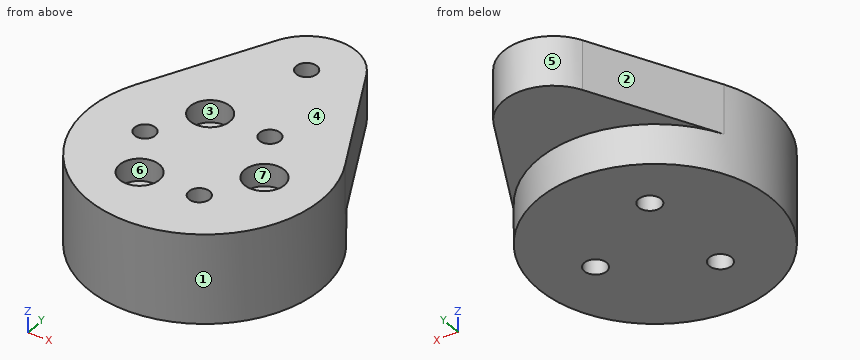
from build123d import *

# Parameters (mm, degrees)
SKETCH1_R           = 23.5
BOSS_EXTRUDE1_DEPTH = 18
BOSS_EXTRUDE2_START = -10
BOSS_EXTRUDE2_DEPTH = 10
SKETCH8_R           = 2.25
CUT_EXTRUDE3_DEPTH  = 50.761933242
SKETCH9_R           = 4
CUT_EXTRUDE4_DEPTH  = 4.5
SKETCH10_R          = 2.1
CUT_EXTRUDE5_DEPTH  = 5.7


with BuildPart() as part:
    # Sketch1 → Boss-Extrude1 (new body)
    with BuildSketch(Plane.XY):
        Circle(SKETCH1_R)
    extrude(amount=BOSS_EXTRUDE1_DEPTH)

    # Sketch7 → Boss-Extrude2 (add)
    with BuildSketch(Plane.XY.offset(18).offset(BOSS_EXTRUDE2_START)):
        with BuildLine():
            ThreePointArc((0, 23.5), (12.323503966, 20.00952898), (20.986171042, 10.575))
            Line((20.986171042, 10.575), (8.93028555, 34.5))
            ThreePointArc((8.93028555, 34.5), (0, 40), (-8.93028555, 34.5))
            Line((-8.93028555, 34.5), (-20.986171042, 10.575))
            ThreePointArc((-20.986171042, 10.575), (-12.323503966, 20.00952898), (0, 23.5))
        make_face()
    extrude(amount=BOSS_EXTRUDE2_DEPTH)

    # Sketch8 → Cut-Extrude3 (cut, through all)
    with BuildSketch(Plane.XY.offset(18)):
        with Locations((12, 0)):
            Circle(SKETCH8_R)
        with Locations((-6, -10.392304845)):
            Circle(SKETCH8_R)
        with Locations((-6, 10.392304845)):
            Circle(SKETCH8_R)
    extrude(amount=-CUT_EXTRUDE3_DEPTH, mode=Mode.SUBTRACT)

    # Sketch9 → Cut-Extrude4 (cut)
    with BuildSketch(Plane.XY.offset(18)):
        with Locations((-6, 10.392304845)):
            Circle(SKETCH9_R)
        with Locations((12, 0)):
            Circle(SKETCH9_R)
        with Locations((-6, -10.392304845)):
            Circle(SKETCH9_R)
    extrude(amount=-CUT_EXTRUDE4_DEPTH, mode=Mode.SUBTRACT)

    # Sketch10 → Cut-Extrude5 (cut)
    with BuildSketch(Plane.XY.offset(18)):
        with Locations((0, 30)):
            Circle(SKETCH10_R)
        with Locations((12, 0)):
            Circle(SKETCH10_R)
        with Locations((6, -10.392304845)):
            Circle(SKETCH10_R)
        with Locations((-6, -10.392304845)):
            Circle(SKETCH10_R)
        with Locations((-12, 0)):
            Circle(SKETCH10_R)
        with Locations((-6, 10.392304845)):
            Circle(SKETCH10_R)
        with Locations((6, 10.392304845)):
            Circle(SKETCH10_R)
    extrude(amount=-CUT_EXTRUDE5_DEPTH, mode=Mode.SUBTRACT)


solid = part.part
Work out the finished part from the listing and answer in its coordinate system (mm). Face numbers are marked on the shaded views. A direction names the side the tool comes from. Give positions to 0.01 mm unless a question says otherwise; leave off trailing zeros. Order: outer loops, then holes, each group sorted by start corner. A loop starts at its lowest first (then second) coordinate and runs counter-clockwise, first axis right, second up. Notation, with made-up numbers: (-1, 40) - (4, 40) arc R20 ccw to (4, 60) - close; hole circle Ø10 at (50, 13.25). An arc over 180 degrees is marked (long way). Answer as CSV lines item,"result". Start each with the question number.
Q1. For the marked faces 1, 2 and 3, determine the directions among +Z, -Z, +X, -X, +Y, -Y from which every point of the face is accessible in a straight line to the end or side of a thin tool.
Q2. The part is cut by section C-C (x = 12). Write down the section's boundary in (y, z).
Q3. Given pin 1 Ø4 at (y, z) = (-8, 2) entering from +X; pin 2 Ø6 at (x, y) = (-6, -10.39) entering from +Z; pin 3 Ø1.5 at (y, z) = (-16.5, 2.5) entering from +X, each flat-ended and moving along its own axis, determine where each tip first touches the part or whether it passes through.
Q4. The part is cut by section D-D (y = 30). Write down the section's boundary in (x, z), then the cut area to 3 significant figures.
Q5. The mould has two halves that part along Y. Classify the marked faces 4, 5, 6 and 7: +Y half, -Y half, draft (parallel to the pull), parting line (faces both ways), or undercut.
Q6. The part is cut by section B-B (x = -6). Write down the section's boundary in (y, z).
Q7. Find the intervals of material crossed by L1, parallel to Y at x = -6, z = 15.3; L2, parallel to Y at x = -6, z = 6.5; L3, parallel to Y at x = -12, z = 16.5, in increasing order. Write a range as [from, to].
Q8. The part is cut by section A-A (y = 0). Write down the section's boundary in (x, z).
Check result:
1,face 1,"-Z"
1,face 2,"+Z, -Z, -X, +Y"
1,face 3,"+Z"
2,outline,"(-20.21, 0) - (-2.25, 0) - (-2.25, 13.5) - (-4, 13.5) - (-4, 18) - (-20.21, 18) - close; (2.25, 0) - (20.21, 0) - (20.21, 8) - (28.41, 8) - (28.41, 18) - (4, 18) - (4, 13.5) - (2.25, 13.5) - close"
3,pin 1,"stops at x = 22.72"
3,pin 2,"stops at z = 13.5"
3,pin 3,"stops at x = 17.44"
4,outline,"(-11.2, 8) - (11.2, 8) - (11.2, 18) - (2.1, 18) - (2.1, 12.3) - (-2.1, 12.3) - (-2.1, 18) - (-11.2, 18) - close"
4,area,"200 mm²"
5,face 4,"draft"
5,face 5,"+Y half"
5,face 6,"undercut"
5,face 7,"undercut"
6,outline,"(-22.72, 0) - (-12.64, 0) - (-12.64, 13.5) - (-14.39, 13.5) - (-14.39, 18) - (-22.72, 18) - close; (-8.14, 0) - (8.14, 0) - (8.14, 13.5) - (6.39, 13.5) - (6.39, 18) - (-6.39, 18) - (-6.39, 13.5) - (-8.14, 13.5) - close; (12.64, 0) - (22.72, 0) - (22.72, 8) - (38, 8) - (38, 18) - (14.39, 18) - (14.39, 13.5) - (12.64, 13.5) - close"
7,L1,"y = [-22.72, -14.39], [-6.39, 6.39], [14.39, 38]"
7,L2,"y = [-22.72, -12.64], [-8.14, 8.14], [12.64, 22.72]"
7,L3,"y = [-20.21, -2.1], [2.1, 28.41]"
8,outline,"(-23.5, 0) - (9.75, 0) - (9.75, 13.5) - (8, 13.5) - (8, 18) - (-9.9, 18) - (-9.9, 12.3) - (-14.1, 12.3) - (-14.1, 18) - (-23.5, 18) - close; (14.25, 0) - (23.5, 0) - (23.5, 18) - (16, 18) - (16, 13.5) - (14.25, 13.5) - close"
